Read the model definition and answer for the solid it produces. Units are mm, in the model's axes. Face numbers are marked on the shaded views. A direction names the side the tool comes from. Coordinates: 2 decimals unless noted, no trailing zeros. Loops run counter-clockwise (first coordinate to the right, second up) from the corner with the lowest first, then second, coordinate; pieces in that order, holes last.
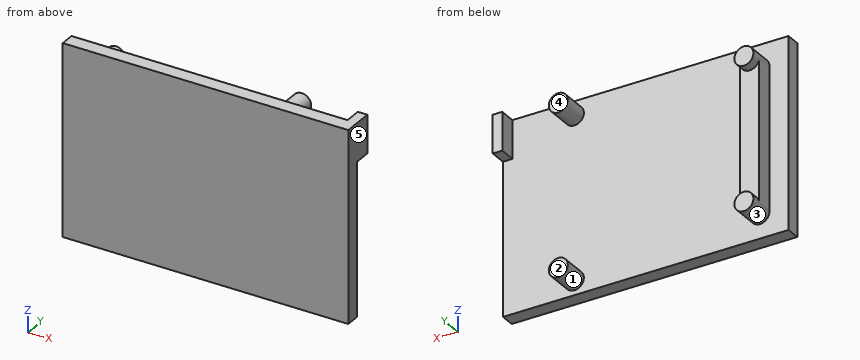
Autodesk Inventor part; units mm, degrees
ref_plane "YZ Plane" through (0, 0, 0) normal (1, 0, 0) x (0, 1, 0)
ref_plane "XZ Plane" through (0, 0, 0) normal (0, 1, 0) x (-1, 0, 0)
ref_plane "XY Plane" through (0, 0, 0) normal (0, 0, 1) x (1, 0, 0)
sketch "Sketch1" plane through (0, 0, 0) normal (0, 1, 0) x (-1, 0, 0)
  line L0 (12.4084, 21.2195) -> (-47.5916, 21.2195)
  line L1 (-47.5916, 21.2195) -> (-47.5916, -18.7805)
  line L2 (-47.5916, -18.7805) -> (12.4084, -18.7805)
  line L3 (12.4084, -18.7805) -> (12.4084, 21.2195)
  circle A0 centre (6.4084, 16.2195) radius 2
  circle A1 centre (6.4084, -13.7805) radius 2
  circle A2 centre (-32.5916, 18.2195) radius 2
  circle A3 centre (-32.5916, -15.7805) radius 2
  line L4 (-47.5916, 21.2195) -> (-47.5916, 0)
  line L5 (-47.5916, 21.2195) -> (-45.5916, 21.2195)
  line L6 (-45.5916, 21.2195) -> (-45.5916, 13.2195)
  line L7 (-45.5916, 13.2195) -> (-47.5916, 13.2195)
  line L8 (-47.5916, 13.2195) -> (-47.5916, 21.2195)
  line L9 (8.4084, -15.7805) -> (4.4084, -15.7805)
  line L10 (4.4084, -15.7805) -> (4.4084, 18.2195)
  line L11 (4.4084, 18.2195) -> (8.4084, 18.2195)
  line L12 (8.4084, 18.2195) -> (8.4084, -15.7805)
  point P0 (0, 0)
  point P1 (8.4084, -13.7805)
  point P2 (8.4084, 16.2195)
  point P3 (4.4084, 16.2195)
  point P4 (4.4084, -13.7805)
  dimension "d0" = 40
  dimension "d1" = 60
  dimension "d2" = 4
  dimension "d3" = 4
  dimension "d4" = 4
  dimension "d5" = 4
  dimension "d6" = 5
  dimension "d7" = 5
  dimension "d9" = 6
  dimension "d10" = 6
  dimension "d11" = 3
  dimension "d12" = 3
  dimension "d13" = 15
  dimension "d14" = 15
  dimension "d15" = 34
  dimension "d16" = 39
  dimension "d17" = 30
  dimension "d26" = 8
  dimension "d27" = 2
extrude "Extrusion1" add sketch "Sketch1" against normal blind 3 contours L3 L2 L1 L7 L6 L0 | L6 L7 L1 L0 | A0 | L12 A1 L10 A0 | A0 L11 L12 | A0 L10 L11 | A1 | L12 L9 A1 | A1 L9 L10 | A2 | A3
extrude "Extrusion2" add sketch "Sketch1" along normal blind 5.5 contours A0 | A1 | A2 | A3
extrude "Extrusion3" add sketch "Sketch1" along normal blind 3.5 contours L6 L7 L1 L0 | L12 A1 L10 A0
properties part number "RFID Reader Frontboard"
Item 1: Find the intervals of material crossed by line 1 along Y through (x, z) = (41, 19.5); line 2 along X through (y, z) = (2, 3), in increasing order.
Numbers:
line 1: y = -3 to 0
line 2: x = -8.41 to -4.41
Item 2: Which of the six approach directions +Z, -Z, +X, -X, +Y, -Y give full straight-line access (tool end or side, diameter ignored) to the marked faces 1 and 2?
Numbers:
face 1: +Y
face 2: +Z, -Z, +X, -X, +Y
Item 3: Given pin 1 (2 mm diameter, centred on x = -7, z = 2.5, fed in from +Y); pin 2 (1.5 mm diameter, centred on x = 32.5, y = 1.5, fed in from +Z); pin 3 (1.8 mm diameter, centred on y = 1, z = 7, fed in from -X), each flat-ended and moving along its own axis, determine where each tip first touches the part or whether it passes through.
Numbers:
pin 1: stops at y = 3.5
pin 2: stops at z = 20.22
pin 3: stops at x = -8.41
Item 4: A cutting plane is placed at C-C on x = -7. Determine the outline of the cut face in (y, z), then the cut area to 3 significant figures.
Numbers:
outline: (-3, -18.78) - (0, -18.78) - (0, -15.69) - (5.5, -15.69) - (5.5, -11.87) - (3.5, -11.87) - (3.5, 14.31) - (5.5, 14.31) - (5.5, 18.13) - (0, 18.13) - (0, 21.22) - (-3, 21.22) - close
area: 254 mm2
Item 5: A cutting plane is placed at A-A on z = 0.5. Determine the outline of the cut face in (x, y).
Numbers:
outline: (-12.41, -3) - (47.59, -3) - (47.59, 0) - (-4.41, 0) - (-4.41, 3.5) - (-8.41, 3.5) - (-8.41, 0) - (-12.41, 0) - close
Item 6: Determine the mould class of the marked faces 3, 4 and 5 for opening direction X: released by +X, released by -X, zero draft, split by the parting line, or undercut.
Numbers:
face 3: undercut
face 4: zero draft
face 5: released by +X
Item 7: A cutting plane is placed at B-B on x = -1. Determine the outline of the cut face in (y, z), then the cut area to 3 significant figures.
Numbers:
outline: (-3, -18.78) - (0, -18.78) - (0, 21.22) - (-3, 21.22) - close
area: 120 mm2
